Can you work these out from the model? Positions are in its coordinate system, mm. A direction names the side the tool comes from. Round coordinates to 2 decimals unless told otherwise and drop trailing zeros. Loops run counter-clockwise (first coordinate to the right, second up) from the corner with the lowest first, then second, coordinate; pieces in that order, holes last. Notation, with made-up numbers: M -10,17 L -4,17 A26 ccw -4,41 Z; hole C -28,34 d4. An arc over 180 degrees is marked long. Return JSON: item names as keys, results as strings.
```python
from build123d import *

# Parameters (mm, degrees)
SKETCH1_R           = 22
SKETCH1_R_2         = 20
BOSS_EXTRUDE1_DEPTH = 180
SKETCH3_W           = 30
SKETCH3_H           = 40
CUT_EXTRUDE1_DEPTH  = 63
BOSS_EXTRUDE2_START = 150
BOSS_EXTRUDE2_DEPTH = 30


with BuildPart() as part:
    # Sketch1 → Boss-Extrude1 (new body)
    with BuildSketch(Plane(origin=(0, 0, 0), x_dir=(1, 0, 0), z_dir=(0, 1, 0))):
        with Locations(Location((0, 0, 0), (0, 0, 90))):
            Circle(SKETCH1_R)
        with Locations(Location((0, 0, 0), (0, 0, 90))):
            Circle(SKETCH1_R_2, mode=Mode.SUBTRACT)
    extrude(amount=BOSS_EXTRUDE1_DEPTH)

    # Sketch3 → Cut-Extrude1 (cut)
    with BuildSketch(Plane(origin=(77.942286341, 45, 0), x_dir=(0.5000000000000041, -0.8660254037844362, 0), z_dir=(0.8660254037844363, 0.5000000000000042, 0))):
        with Locations((-155.884572681, 0)):
            Rectangle(SKETCH3_W, SKETCH3_H)
    extrude(amount=-CUT_EXTRUDE1_DEPTH, mode=Mode.SUBTRACT)

    # Sketch1<3> → Boss-Extrude2 (add)
    with BuildSketch(Plane(origin=(0, 0, 0), x_dir=(1, 0, 0), z_dir=(0, 1, 0)).offset(BOSS_EXTRUDE2_START)):
        with BuildLine():
            ThreePointArc((20, 0), (14.142135624, -14.142135624), (0, -20))
            Line((0, -20), (0, -22))
            ThreePointArc((0, -22), (15.556349186, -15.556349186), (22, 0))
            ThreePointArc((22, 0), (15.556349186, 15.556349186), (0, 22))
            Line((0, 22), (0, 20))
            ThreePointArc((0, 20), (14.142135624, 14.142135624), (20, 0))
        make_face()
    extrude(amount=BOSS_EXTRUDE2_DEPTH)


solid = part.part
```
Q1. Suppose I cut it at C-C, the plane y = 89. Please give me the cut outline in (x, z), plus the area to 3 significant figures.
Results:
{"outline": "C 0,0 d44; hole C 0,0 d40", "area": "264 mm2"}
Q2. Suppose I cut it at D-D, the plane z = 4. Please give me the cut outline in (x, y), plus the area to 3 significant figures.
Results:
{"outline": "M -21.63,0 L -19.6,0 L -19.6,151.37 L -21.63,150.19 Z; M 19.6,0 L 21.63,0 L 21.63,180 L 19.6,180 Z", "area": "674 mm2"}
Q3. On a 3-axis mill with a long thin cutter (end or side, diameter ignored), from which of +Z, -Z, +X, -X, +Y, -Y can I reach the whole of each face in a straight line? I mean faces 3 (the flat face through (-6, 171, 20)), 4 (the flat face through (18, 0, -10)). Say none if no direction works.
Results:
{"face 3": "-X, +Y", "face 4": "+Z, -Z, +X, -X, -Y"}
Q4. I'm going to push flat-ended pins straight in: pin 1 Ø10 at (y, z) = (91.5, 15) entering from -X; pin 2 Ø1 at (x, y) = (15, 148) entering from -Z; pin 3 Ø1 at (y, z) = (34, -17.5) entering from +X; pin 4 Ø24 at (x, z) = (0, 0) entering from -Y. Where does each tip first touch, or does it pass through?
Results:
{"pin 1": "stops at x = -19.6", "pin 2": "stops at z = -16.55", "pin 3": "stops at x = 13.96", "pin 4": "passes through"}
Q5. Thinking about a two-plate mould opening in Z: for faces 1 (the flat face through (-6, 171, -20)), 2 (the flat face through (20.2, 180, 0.1)), which applies, pulls with the +Z half, pulls with the -Z half, needs draft (parallel to the pull), parting line crosses it, or undercut?
Results:
{"face 1": "undercut", "face 2": "needs draft"}
Q6. Suppose I cut it at A-A, the plane x = -3. Please give me the cut outline in (y, z).
Results:
{"outline": "M 0,-21.79 L 180,-21.79 L 180,-20 L 160.95,-20 L 160.95,-19.77 L 0,-19.77 Z; M 0,19.77 L 160.95,19.77 L 160.95,20 L 180,20 L 180,21.79 L 0,21.79 Z"}
Q7. If I drill on line 1 along X through (y, z) = (50, 0); line 2 along X through (y, z) = (107.5, 13); line 3 along Z through (x, y) = (-2, 104), over which ranges is the centre line in solid material (lowest first)?
Results:
{"line 1": "x = -22 to -20, 20 to 22", "line 2": "x = -17.75 to -15.2, 15.2 to 17.75", "line 3": "z = -21.91 to -19.9, 19.9 to 21.91"}
Q8. Suppose I cut it at B-B, the plane z = 13. Please give me the cut outline in (x, y), plus the area to 3 significant figures.
Results:
{"outline": "M -17.75,0 L -15.2,0 L -15.2,153.9 L -17.75,152.43 Z; M 15.2,0 L 17.75,0 L 17.75,180 L 15.2,180 Z", "area": "849 mm2"}
